Verification items for this drawing (mm, ordinates from the low corner). A direction names the side the tool comes from. Coordinates: 2 decimals unless noted, no trailing zeros. Loops run counter-clockwise (first coordinate to the right, second up) from the corner with the lowest first, then second, coordinate; pieces in that order, holes last. Notation, with made-up numbers: M -13,50.5 L 11,50.5 A19 ccw 11,75.5 Z; hole C 33,-27 d7. An arc over 180 degrees is marked long. Return JSON: item names as keys, results as strings.
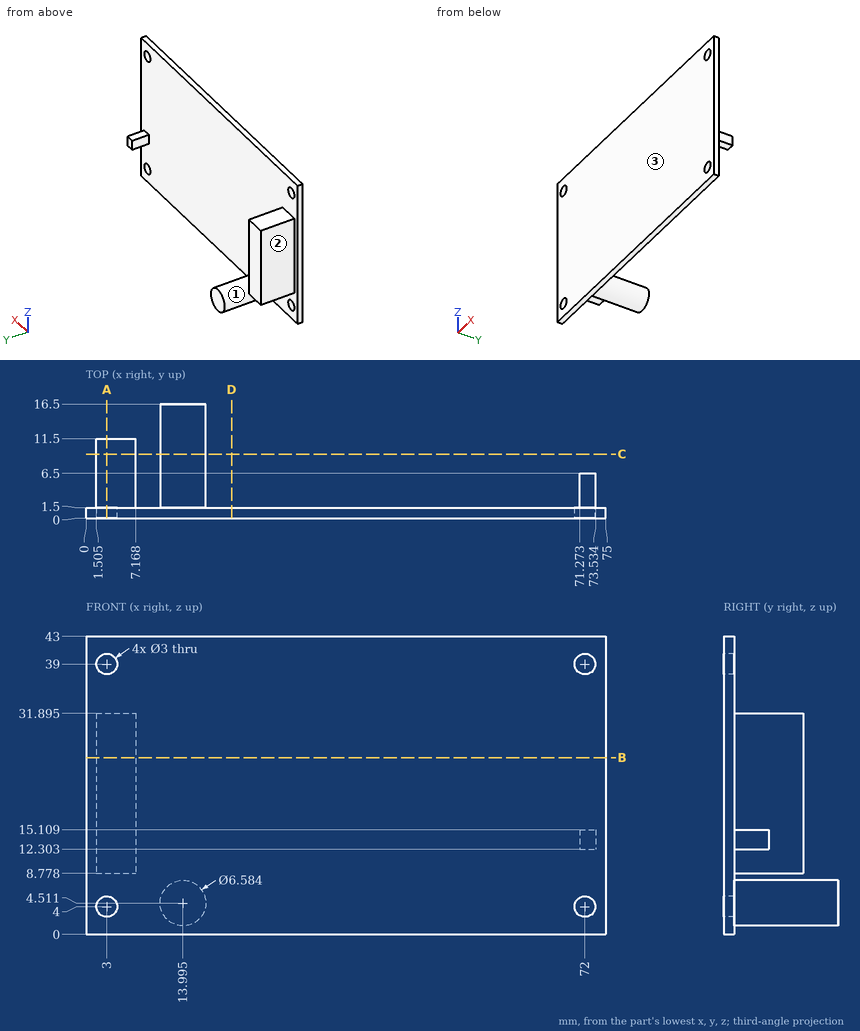
1) Scan lines: line 1 along X through (y, z) = (1.15, 39); line 2 along Z through (x, y) = (3, 0.8); line 3 along X through (y, z) = (2.5, 12.5) (1 decimal). Record each from-to range of solid material in increasing order. Write a range as [from, to].
Answers:
{"line 1": "[0, 1.5], [4.5, 70.5], [73.5, 75]", "line 2": "[0, 2.5], [5.5, 37.5], [40.5, 43]", "line 3": "[1.5, 7.2], [71.3, 73.5]"}
2) Section check B-B on z = 25.5. Record the cut outline in (x, y) (1 decimal), then the cut area to 3 significant figures.
Answers:
{"outline": "M 0,0 L 75,0 L 75,1.5 L 7.2,1.5 L 7.2,11.5 L 1.5,11.5 L 1.5,1.5 L 0,1.5 Z", "area": "169 mm²"}
3) Section check A-A on x = 3. Record the cut outline in (y, z) (1 decimal).
Answers:
{"outline": "M 0,0 L 1.5,0 L 1.5,2.5 L 0,2.5 Z; M 0,5.5 L 1.5,5.5 L 1.5,8.8 L 11.5,8.8 L 11.5,31.9 L 1.5,31.9 L 1.5,37.5 L 0,37.5 Z; M 0,40.5 L 1.5,40.5 L 1.5,43 L 0,43 Z"}
4) Section check D-D on x = 21. Record the cut outline in (y, z).
Answers:
{"outline": "M 0,0 L 1.5,0 L 1.5,43 L 0,43 Z"}
5) Set-up check for the marked faces 1, 2 and 3: record each of +Z, -Z, +X, -X, +Y, -Y from which the full face is reachable in a straight line by a thin tool's end or side.
Answers:
{"face 1": "+Y", "face 2": "+Z, -Z, -X, +Y", "face 3": "+Z, -Z, +X, -X, -Y"}
6) Go/stop test with flat-tipped pins: pin 1 Ø6 at (x, z) = (16, 18) entering from +Y; pin 2 Ø6 at (x, y) = (5.5, 5.5) entering from +Z (1 decimal); pin 3 Ø0.7 at (x, y) = (73, 4) entering from -Z. Record where each tip stops, or that it passes through.
Answers:
{"pin 1": "y = 1.5", "pin 2": "z = 31.9", "pin 3": "z = 12.3"}
7) Section check C-C on y = 9.25. Record the cut outline in (x, z) (1 decimal).
Answers:
{"outline": "M 1.5,8.8 L 7.2,8.8 L 7.2,31.9 L 1.5,31.9 Z; C 14,4.5 d6.6"}
